```python
from build123d import *

# Parameters (mm, degrees)
F1_DEPTH = 25.4


with BuildPart() as f1:
    # F0 (on Top) → F1 (new body)
    with BuildSketch(Plane.XY):
        with BuildLine():
            Line((0, 12.7), (0, 0))
            Line((0, 0), (12.7, 0))
            Line((12.7, 0), (12.7, 6.35))
            ThreePointArc((12.7, 6.35), (10.8401280605, 10.8401280605), (6.35, 12.7))
            Line((6.35, 12.7), (0, 12.7))
        make_face()
        with BuildLine():
            Line((12.7, 6.35), (12.7, 0))
            Line((12.7, 0), (38.1, 0))
            ThreePointArc((38.1, 0), (31.75, 6.35), (38.1, 12.7))
            Line((38.1, 12.7), (23.6217547208, 12.7))
            Line((23.6217547208, 12.7), (18.1608773604, 12.7))
            Line((18.1608773604, 12.7), (12.7, 12.7))
            Line((12.7, 12.7), (12.7, 6.35))
        make_face()
        with BuildLine():
            Line((0, 38.1), (0, 12.7))
            Line((0, 12.7), (6.35, 12.7))
            Line((6.35, 12.7), (12.7, 12.7))
            Line((12.7, 12.7), (12.7, 19.05))
            Line((12.7, 19.05), (12.7, 38.1))
            ThreePointArc((12.7, 38.1), (6.35, 31.75), (0, 38.1))
        make_face()
        with BuildLine():
            ThreePointArc((38.1, 12.7), (31.75, 6.35), (38.1, 0))
            Line((38.1, 0), (38.1, 12.7))
        make_face()
        with BuildLine():
            Line((38.1, 12.7), (38.1, 0))
            ThreePointArc((38.1, 0), (42.5901280605, 1.8598719395), (44.45, 6.35))
            ThreePointArc((44.45, 6.35), (42.5901280605, 10.8401280605), (38.1, 12.7))
        make_face()
        with BuildLine():
            ThreePointArc((6.35, 12.7), (10.8401280605, 10.8401280605), (12.7, 6.35))
            Line((12.7, 6.35), (12.7, 12.7))
            Line((12.7, 12.7), (6.35, 12.7))
        make_face()
        with BuildLine():
            ThreePointArc((12.7, 38.1), (6.35, 44.45), (0, 38.1))
            Line((0, 38.1), (12.7, 38.1))
        make_face()
        with BuildLine():
            Line((12.7, 38.1), (0, 38.1))
            ThreePointArc((0, 38.1), (6.35, 31.75), (12.7, 38.1))
        make_face()
    extrude(amount=F1_DEPTH)


solid = f1.part
```
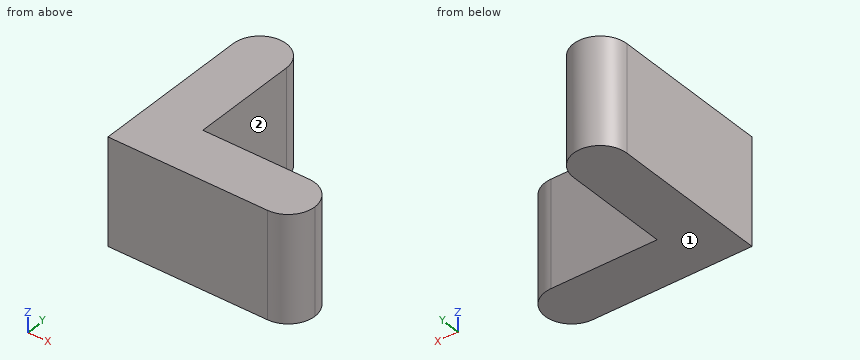
The listing builds one solid part. Answer for the finished solid, in the listing's coordinates (mm). Face numbers are marked on the shaded views. A direction names the side the tool comes from. Coordinates: 2 decimals unless noted, no trailing zeros. Loops run counter-clockwise (first coordinate to the right, second up) from the corner with the lowest first, then second, coordinate; pieces in that order, holes last. Notation, with made-up numbers: (-24, 44.5) -> (-17, 44.5) arc R21 cw to (-17, 72.5) -> close; hole circle Ø6 at (-18.5, -18.75). An arc over 180 degrees is marked (long way). Use one line per item in the form item = value. Start each with the question number.
Item 1: Consider L1, parallel to X at y = 30, z = 22.75; L2, parallel to Y at x = 10.5, z = 8.75. Determine where each line is inside the solid, lowest interval first. Write a range as [from, to].
Item 2: Flat-ended cylindrical pins translate along their axes: pin 1 Ø12 at (x, y) = (23.5, 39) entering from +Z; pin 2 Ø3 at (y, z) = (35, 19) entering from +X; pin 3 Ø8 at (y, z) = (13.5, 6.5) entering from +X. Find the tip coordinate at first contact, or state that the pin passes through.
Item 3: The part is cut by section B-B on x = 17.5. Determine the outline of the cut face in (y, z), then the cut area to 3 significant figures.
Item 4: A tool of negligible diameter and unlimited length cuts with its end or side. For the marked faces 1 and 2, from which of +Z, -Z, +X, -X, +Y, -Y can it reach the whole face along a straight path? Write none if from no direction.
Item 5: The part is cut by section A-A on z = 5.75. Determine the outline of the cut face in (x, y).
Answer key:
q1.L1 = [0, 12.7]
q1.L2 = [0, 42.91]
q2.pin_1 = through
q2.pin_2 = 12.7
q2.pin_3 = 43.61
q3.outline = (0, 0) -> (12.7, 0) -> (12.7, 25.4) -> (0, 25.4) -> close
q3.area = 323 mm2
q4.face_1 = -Z, +X, -X, +Y, -Y
q4.face_2 = +Z, -Z, +X, +Y
q5.outline = (0, 0) -> (38.1, 0) arc R6.35 ccw to (38.1, 12.7) -> (12.7, 12.7) -> (12.7, 38.1) arc R6.35 ccw to (0, 38.1) -> close
